```python
from build123d import *

# Parameters (mm, degrees)
SKETCH_1_W            = 10
SKETCH_1_H            = 10
EXTRUDE_1_DEPTH       = 28
SKETCH_2_R            = 4.499999995
CUT_EXTRUDE_2_DEPTH   = 31.149626863
SKETCH_3_R            = 1.5
CUT_EXTRUDE_1_DEPTH   = 31.149626863
SKETCH_4_R            = 1.999999994
CUT_EXTRUDE_2_2_DEPTH = 31.149626863


with BuildPart() as part:
    # Эскиз1 → Вытянуть1 (new body)
    with BuildSketch(Plane(origin=(0, 0, 0), x_dir=(1, 0, 0), z_dir=(0, 1, 0))):
        Rectangle(SKETCH_1_W, SKETCH_1_H)
    extrude(amount=EXTRUDE_1_DEPTH)

    # Эскиз2 → Cut-Extrude 2 (cut, through all)
    with BuildSketch(Plane.XY.offset(5)):
        with Locations((5.000000005, 10.000000001)):
            Circle(SKETCH_2_R)
    extrude(amount=-CUT_EXTRUDE_2_DEPTH, mode=Mode.SUBTRACT)

    # Эскиз3 → Вырез-Вытянуть1 (cut, through all)
    with BuildSketch(Plane(origin=(5, 0, 0), x_dir=(0, 0, -1), z_dir=(1, 0, 0))):
        with Locations((0, 3.309697202)):
            Circle(SKETCH_3_R)
        with Locations((0, 18.798896008)):
            Circle(SKETCH_3_R)
    extrude(amount=-CUT_EXTRUDE_1_DEPTH, mode=Mode.SUBTRACT)

    # Эскиз4 → Cut-Extrude 2 2 (cut, through all)
    with BuildSketch(Plane.XY.offset(5)):
        with Locations((4.999999971, 22.940656165)):
            Circle(SKETCH_4_R)
    extrude(amount=-CUT_EXTRUDE_2_2_DEPTH, mode=Mode.SUBTRACT)


solid = part.part
```
Input: part model. Units: mm. Frame: model coordinates. Give positions to 0.01 mm unless a question says otherwise; leave off trailing zeros. Order: outer loops, then holes, each group sorted by start corner. A loop starts at its lowest first (then second) coordinate and runs counter-clockwise, first axis right, second up. Notation, with made-up numbers: (-10.75, 12) - (23.25, 12) arc R22 cw to (23.25, 44) - close; hole circle Ø10 at (81, 0). An arc over 180 degrees is marked (long way). One line per item, written item: value.
1. Cut plane B-B, the plane x = 4.25. Output: boundary loops of the cut face in (y, z), and give its area (3 significant figures).
Determined:
outline: (0, -5) - (5.56, -5) - (5.56, 5) - (0, 5) - close; (14.44, -5) - (21.09, -5) - (21.09, 5) - (14.44, 5) - close; (24.79, -5) - (28, -5) - (28, 5) - (24.79, 5) - close; hole circle Ø3 at (3.31, 0); hole circle Ø3 at (18.8, 0)
area: 140 mm2
2. Cut plane C-C, the plane y = 4.25. Output: boundary loops of the cut face in (x, z).
Determined:
outline: (-5, -5) - (5, -5) - (5, -1.17) - (-5, -1.17) - close; (-5, 1.17) - (5, 1.17) - (5, 5) - (-5, 5) - close
3. Cut plane D-D, the plane z = -3. Output: boundary loops of the cut face in (x, y).
Determined:
outline: (-5, 0) - (5, 0) - (5, 5.5) arc R4.5 cw to (5, 14.5) - (5, 20.94) arc R2 cw to (5, 24.94) - (5, 28) - (-5, 28) - close
4. Cut plane A-A, the plane z = 0. Output: boundary loops of the cut face in (x, y), and give its area (3 significant figures).
Determined:
outline: (-5, 0) - (5, 0) - (5, 1.81) - (-5, 1.81) - close; (-5, 4.81) - (5, 4.81) - (5, 5.5) arc R4.5 cw to (5, 14.5) - (5, 17.3) - (-5, 17.3) - close; (-5, 20.3) - (5, 20.3) - (5, 20.94) arc R2 cw to (5, 24.94) - (5, 28) - (-5, 28) - close
area: 182 mm2
5. Line query: probe 1 along Y at (x, z) = (-3, 0); probe 2 along Y at (x, z) = (-4, -0.5); probe 3 along Y at (x, z) = (2, 0). Output: solid intervals per line, ascending.
Determined:
probe 1: 0 to 1.81, 4.81 to 17.3, 20.3 to 28
probe 2: 0 to 1.9, 4.72 to 17.38, 20.21 to 28
probe 3: 0 to 1.81, 4.81 to 6.65, 13.35 to 17.3, 20.3 to 28
6. Pin query (flat end, axial travel): pin 1 Ø1.5 at (y, z) = (11, 3) entering from +X. Return the tip coordinate at first contact, or that it passes through.
Determined:
pin 1: x = 0.85
7. Draft query along Y for faces 1 (the face through (0.5, 10.1, 0.1)), 2 (the face through (0, 28, 0)), 3 (the face through (5, 1, 0)). Return one class per face: released by +Y, released by -Y, zero draft, split by the parting line, or undercut.
Determined:
face 1: undercut
face 2: released by +Y
face 3: zero draft
